```python
from build123d import *

# Parameters (mm, degrees)
F0_W     = 43.5
F0_H     = 12
F1_DEPTH = 1
F2_W     = 8.8
F2_H     = 6.7
F3_DEPTH = 3.5
F4_R     = 1
F5_R     = 0.3


with BuildPart() as f1:
    # F0 (on Top) → F1 (new body)
    with BuildSketch(Plane.XY):
        with Locations((-4.144736, 0.530427)):
            Rectangle(F0_W, F0_H)
    extrude(amount=F1_DEPTH)

    # F2 (on face) → F3 (join)
    with BuildSketch(Plane.XY.offset(1)):
        with Locations((-17.094736, 0.480427)):
            Rectangle(F2_W, F2_H)
        with BuildLine():
            Line((-21.494736, -2.869573), (-21.494736, 3.830427))
            ThreePointArc((-21.494736, 3.830427), (-24.844736, 0.480427), (-21.494736, -2.869573))
        make_face()
        with BuildLine():
            ThreePointArc((-12.694736, -2.869573), (-9.344736, 0.480427), (-12.694736, 3.830427))
            Line((-12.694736, 3.830427), (-12.694736, -2.869573))
        make_face()
        with BuildLine():
            Line((12.305264, 3.830427), (3.505264, 3.830427))
            ThreePointArc((3.505264, 3.830427), (0.155264, 0.480427), (3.505264, -2.869573))
            Line((3.505264, -2.869573), (12.305264, -2.869573))
            ThreePointArc((12.305264, -2.869573), (15.655264, 0.480427), (12.305264, 3.830427))
        make_face()
    extrude(amount=F3_DEPTH)

    # F4
    f4_edges = [f1.edges().sort_by_distance(p)[0] for p in [
        (-25.894736, -5.469573, 0.5),
        (17.605264, 6.530427, 0.5),
        (17.605264, -5.469573, 0.5),
        (-25.894736, 6.530427, 0.5),
    ]]
    fillet(f4_edges, radius=F4_R)

    # F5
    f5_edges = [f1.edges().sort_by_distance(p)[0] for p in [
        (-17.094736, 3.830427, 4.5),
        (7.905264, 3.830427, 4.5),
    ]]
    fillet(f5_edges, radius=F5_R)


solid = f1.part
```
Work out the finished part from the listing and answer in its coordinate system (mm). A direction names the side the tool comes from. Coordinates: 2 decimals unless noted, no trailing zeros. Loops run counter-clockwise (first coordinate to the right, second up) from the corner with the lowest first, then second, coordinate; pieces in that order, holes last.
1) Section A-A (z = 3.6) is taken. Give the vertices of the cut face in (x, y).
Results:
outline: (-21.49, -2.87) - (-12.69, -2.87) arc R3.35 ccw to (-12.69, 3.83) - (-21.49, 3.83) arc R3.35 ccw to start; (3.51, -2.87) - (12.31, -2.87) arc R3.35 ccw to (12.31, 3.83) - (3.51, 3.83) arc R3.35 ccw to start
2) Section C-C (y = 4.5) is taken. Give the vertices of the cut face in (x, z), plus the area to 3 significant figures.
Results:
outline: (-25.89, 0) - (17.61, 0) - (17.61, 1) - (-25.89, 1) - close
area: 43.5 mm2
3) Section B-B (x = -16) is taken. Give the vertices of the cut face in (y, z).
Results:
outline: (-5.47, 0) - (6.53, 0) - (6.53, 1) - (3.83, 1) - (3.83, 4.2) arc R0.3 ccw to (3.53, 4.5) - (-2.57, 4.5) arc R0.3 ccw to (-2.87, 4.2) - (-2.87, 1) - (-5.47, 1) - close
4) Flat-ended cylindrical pins translate along their axes: pin 1 (1.6 mm diameter, centred on x = -17, z = 2, fed in from -Y); pin 2 (1.6 mm diameter, centred on x = -19, z = 2.5, fed in from +Y); pin 3 (1 mm diameter, centred on y = 4, z = 4, fed in from -X). Find the tip coordinate at first contact, or state that the pin passes through.
Results:
pin 1: stops at y = -2.87
pin 2: stops at y = 3.83
pin 3: stops at x = -22.95
5) For a pull along X with two mould halves and no side action, classify faces 6 (the cylindrical face through (-9.346, 0.407, 2.578)), 7 (the flat face through (-4.4, 6.53, 0.5)), 8 (the cylindrical face through (17.3, 6.25, 0.51)) as +X half, -X half, draft (parallel to the pull), parting line (faces both ways), or undercut.
Results:
face 6: undercut
face 7: draft
face 8: +X half
6) Section D-D (x = -6) is taken. Give the vertices of the cut face in (y, z), plus the area to 3 significant figures.
Results:
outline: (-5.47, 0) - (6.53, 0) - (6.53, 1) - (-5.47, 1) - close
area: 12.0 mm2
7) For faces 1 (the flat face through (-4, 1, 1)), 2 (the flat face through (8, 3.83, 3)), 3 (the cylindrical face through (-24.844, 0.554, 2.578)), 4 (the flat face through (-17, -2.87, 3)), 5 (the cylindrical face through (15.654, 0.407, 2.578)), determine the directions among +Z, -Z, +X, -X, +Y, -Y from which every point of the face is accessible in a straight line to the end or side of a thin tool.
Results:
face 1: +Z
face 2: +Z, +X, -X, +Y
face 3: +Z, -X
face 4: +Z, +X, -X, -Y
face 5: +Z, +X
8) Consider probe 1 along Z at (x, y) = (-24, -4.25); probe 2 along X at (y, z) = (-2, 3.75); probe 3 along Y at (x, z) = (-13, 4.25). Determine where each line is inside the solid, lowest interval first.
Results:
probe 1: z = 0 to 1
probe 2: x = -23.75 to -10.44, 1.25 to 14.56
probe 3: y = -2.87 to 3.83
